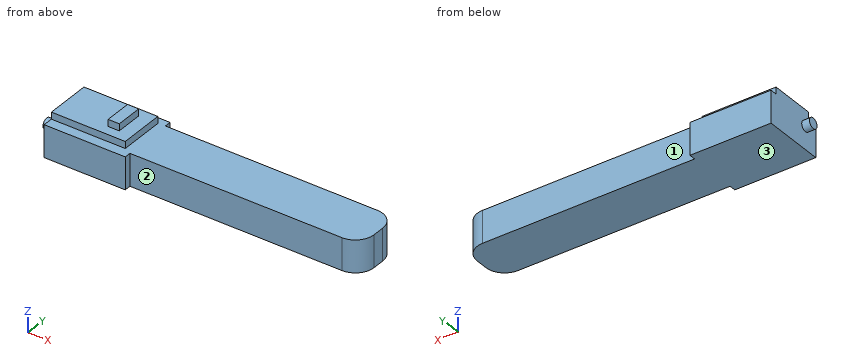
```python
from build123d import *

# Parameters (mm, degrees)
F1_DEPTH = 26.162
F2_R     = 4.242227
F3_DEPTH = 6.35
F5_DEPTH = 5.588
F6_W     = 9.096682
F6_H     = 22.018083
F7_DEPTH = 5.588
F8_R     = 15.24


with BuildPart() as f1:
    # F0 (on Top) → F1 (new body)
    with BuildSketch(Plane.XY):
        Polygon((-127, -25.4), (-60.96, -25.4), (-60.96, -20.1168), (127, -20.1168), (127, 20.1168), (-60.96, 20.1168), (-60.96, 25.4), (-127, 25.4), align=None)
    extrude(amount=F1_DEPTH)

    # F2 (on face) → F3 (join)
    with BuildSketch(Plane(origin=(-127, 0, 0), x_dir=(0, -1, 0), z_dir=(-1, 0, 0))):
        with Locations((13.661651, 18.503753)):
            Circle(F2_R)
    extrude(amount=F3_DEPTH)

    # F4 (on face) → F5 (join)
    with BuildSketch(Plane.XY.offset(26.162)):
        Polygon((-66.817649, 19.667143), (-127, 19.667143), (-127, -17.230507), (-66.817649, -17.230507), (-66.817649, 1.218318), align=None)
    extrude(amount=F5_DEPTH)

    # F6 (on face) → F7 (join)
    with BuildSketch(Plane.XY.offset(31.75)):
        with Locations((-81.979908, 1.763641)):
            Rectangle(F6_W, F6_H)
    extrude(amount=F7_DEPTH)

    # F8
    f8_edges = [f1.edges().sort_by_distance(p)[0] for p in [
        (127, -20.1168, 13.081),
        (127, 20.1168, 13.081),
    ]]
    fillet(f8_edges, radius=F8_R)


solid = f1.part
```
Geometry check sheet. Reference: the model listing, model coordinates, mm. Face numbers are marked on the shaded views. A direction names the side the tool comes from. Coordinates: 2 decimals unless noted, no trailing zeros. Order: outer loops, then holes, each group sorted by start corner. A loop starts at its lowest first (then second) coordinate and runs counter-clockwise, first axis right, second up.
Item 1: Depth check by flat-ended pin: pin 1 (1.7 mm diameter, centred on y = 6.5, z = 29.5, fed in from +X); pin 2 (1 mm diameter, centred on y = -16, z = 5.5, fed in from -X); pin 3 (2 mm diameter, centred on y = -15.5, z = 24, fed in from +X). Enter the tip coordinate at first touch or a pass-through.
Item 2: Section check D-D (x = -80). Enter the section's corners in (y, z).
Item 3: Section check C-C (z = 28.5). Enter the section's corners in (x, y).
Item 4: Section check A-A (y = 2.5). Enter the section's corners in (x, z), plus the area to 3 significant figures.
Item 5: Scan lines: line 1 along X through (y, z) = (14, 27); line 2 along Z through (x, y) = (72.5, -12); line 3 along Z through (x, y) = (-121, 3). Record each from-to range of solid material in increasing order.
Item 6: Section check B-B (x = -116). Enter the section's corners in (y, z), plus the area to 3 significant figures.
Item 7: Tool access check on the marked faces 1, 2 and 3. Record the directions out of +Z, -Z, +X, -X, +Y, -Y that give a thin tool (end or side, any length) a straight path to the whole face; none if there is none.
Check sheet entries:
1. pin 1: stops at x = -66.82
1. pin 2: stops at x = -127
1. pin 3: stops at x = 123.58
2. outline: (-25.4, 0) - (25.4, 0) - (25.4, 26.16) - (19.67, 26.16) - (19.67, 31.75) - (12.77, 31.75) - (12.77, 37.34) - (-9.25, 37.34) - (-9.25, 31.75) - (-17.23, 31.75) - (-17.23, 26.16) - (-25.4, 26.16) - close
3. outline: (-127, -17.23) - (-66.82, -17.23) - (-66.82, 19.67) - (-127, 19.67) - close
4. outline: (-127, 0) - (127, 0) - (127, 26.16) - (-66.82, 26.16) - (-66.82, 31.75) - (-77.43, 31.75) - (-77.43, 37.34) - (-86.53, 37.34) - (-86.53, 31.75) - (-127, 31.75) - close
4. area: 7,030 mm2
5. line 1: x = -127 to -66.82
5. line 2: z = 0 to 26.16
5. line 3: z = 0 to 31.75
6. outline: (-25.4, 0) - (25.4, 0) - (25.4, 26.16) - (19.67, 26.16) - (19.67, 31.75) - (-17.23, 31.75) - (-17.23, 26.16) - (-25.4, 26.16) - close
6. area: 1,540 mm2
7. face 1: +Z, -Z, +X, +Y
7. face 2: +Z, -Z, +X, -Y
7. face 3: -Z, +X, -X, +Y, -Y
